Input: part model. Units: mm. Frame: model coordinates. A direction names the side the tool comes from. Give positions to 0.01 mm unless a question says otherwise; leave off trailing zeros. Loops run counter-clockwise (first coordinate to the right, second up) from the corner with the lowest first, then second, coordinate; pieces in that order, holes last. Notation, with made-up numbers: M 7.25,-27.75 L 31.25,-27.75 A7 ccw 31.25,-23.75 Z; hole C 56.25,54.5 d10. An arc over 180 degrees is marked long. Use CSV: the item, a comma, the result in double quotes. Start each with the question number.
from build123d import *

# Parameters (mm, degrees)
BOSS_EXTRUDE1_DEPTH = 73
FILLET1_R           = 0.2


with BuildPart() as part:
    # Sketch1 → Boss-Extrude1 (new body)
    with BuildSketch(Plane(origin=(0, 0, 0), x_dir=(1, 0, 0), z_dir=(0, 1, 0))):
        Polygon((0, 0), (54.275908818, 0), (54.275908818, 22), (44.720772546, 27.516660498), (31.720772546, 5), (0, 19.791639161), align=None)
    extrude(amount=BOSS_EXTRUDE1_DEPTH)

    # Fillet1
    fillet1_edges = [part.edges().sort_by_distance(p)[0] for p in [
        (31.720772546, 36.5, -5),
        (44.720772546, 36.5, -27.516660498),
        (54.275908818, 36.5, -22),
        (0, 36.5, -19.791639161),
        (54.275908818, 73, -11),
        (49.498340682, 73, -24.758330249),
        (38.220772546, 73, -16.258330249),
        (15.860386273, 73, -12.39581958),
        (38.220772546, 0, -16.258330249),
        (49.498340682, 0, -24.758330249),
        (54.275908818, 0, -11),
        (0, 73, -9.89581958),
        (0, 0, -9.89581958),
        (15.860386273, 0, -12.39581958),
    ]]
    fillet(fillet1_edges, radius=FILLET1_R)


solid = part.part
Item 1: First-contact query: pin 1 Ø4 at (x, y) = (25, 23.5) entering from -Z; pin 2 Ø1 at (x, z) = (38, -17.5) entering from +Y. Flat tips, straight axial feed; report the tip coordinate or a pass-through.
Item 2: Section A-A (y = 29.5). Output: boundary loops of the cut face in (x, z), then the cut area to 3 significant figures.
Item 3: Material intervals for line 1 (X direction, y = 11, z = -12.5); line 2 (X direction, y = 67.5, z = -12.75); line 3 (X direction, y = 24, z = -22), sorted ascending.
Item 4: Set-up query: faces 1 (the cylindrical face through (38.18, 0.06, -16.07)), 2 (the flat face through (38.31, 35.99, -16.41)), 3 (the flat face through (27, 73, -5)), 4 (the cylindrical face through (38.18, 72.94, -16.07)), 5 (the flat face through (27, 36, 0)). Return all of +Z, -Z, +X, -X, +Y, -Y with unobstructed straight access to the full face (end or side cutting, diameter ignored); none if empty.
Recorded:
1,pin 1,"z = -9.07"
1,pin 2,"through"
2,outline,"M 0,-19.48 A0.2 ccw 0.28,-19.66 L 31.55,-5.08 A0.2 cw 31.81,-5.16 L 44.62,-27.34 A0.2 ccw 44.89,-27.42 L 54.18,-22.06 A0.2 ccw 54.28,-21.88 L 54.28,0 L 0,0 Z"
2,area,"841 mm²"
3,line 1,"0 to 15.64, 36.05 to 54.28"
3,line 2,"0 to 15.1, 36.2 to 54.28"
3,line 3,"41.54 to 54.24"
4,face 1,"-Z, -Y"
4,face 2,"-Z, +Y, -Y"
4,face 3,"+Z, -Z, +X, -X, +Y"
4,face 4,"-Z, +Y"
4,face 5,"+Z, +X, -X, +Y, -Y"
